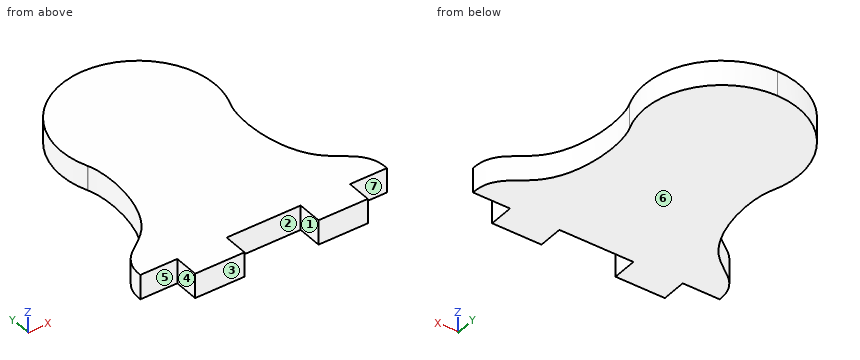
```python
from build123d import *

# Parameters (mm, degrees)
BOSS_EXTRUDE1_DEPTH = 4


with BuildPart() as part:
    # Sketch1 → Boss-Extrude1 (new body)
    with BuildSketch(Plane.XY):
        with BuildLine():
            Line((-6, 0), (0, 0))
            Line((0, 0), (0, 40.631746277))
            ThreePointArc((0, 40.631746277), (-10.364472675, 35.119428737), (-11.587783027, 23.444179263))
            ThreePointArc((-11.587783027, 23.444179263), (-11.580453389, 23.426100806), (-11.573095546, 23.40803381))
            add(Edge.make_bspline(
                [(-20, 0), (-20.119909127, 4.314498585), (-10.868715854, 6.603153145), (-10.177575907, 19.938030034), (-11.573095546, 23.40803381)],
                knots=[0, 0, 0, 0, 0.217805144, 0.603787586, 0.603787586, 0.603787586, 0.603787586], degree=3))
            Line((-20, 0), (-14, 0))
            Line((-14, 0), (-14, -4))
            Line((-14, -4), (-6, -4))
            Line((-6, -4), (-6, 0))
        make_face()
        with BuildLine():
            Line((0, 40.631746277), (0, 0))
            Line((0, 0), (6, 0))
            Line((6, 0), (6, -4))
            Line((6, -4), (14, -4))
            Line((14, -4), (14, 0))
            Line((14, 0), (20, 0))
            add(Edge.make_bspline(
                [(20, 0), (20.119909127, 4.314498585), (10.868715854, 6.603153145), (10.177575907, 19.938030034), (11.573095546, 23.40803381)],
                knots=[0, 0, 0, 0, 0.217805144, 0.603787586, 0.603787586, 0.603787586, 0.603787586], degree=3))
            ThreePointArc((11.573095546, 23.40803381), (11.580453389, 23.426100806), (11.587783027, 23.444179263))
            ThreePointArc((11.587783027, 23.444179263), (10.364472675, 35.119428737), (0, 40.631746277))
        make_face()
    extrude(amount=BOSS_EXTRUDE1_DEPTH)


solid = part.part
```
Input: part model. Units: mm. Frame: model coordinates. Face numbers are marked on the shaded views. A direction names the side the tool comes from. Coordinates: 2 decimals unless noted, no trailing zeros. Loops run counter-clockwise (first coordinate to the right, second up) from the corner with the lowest first, then second, coordinate; pieces in that order, holes last. Notation, with made-up numbers: M 67.25,62 L 114.25,62 A36 cw 114.25,97 Z; hole C 43,68 d3. An arc over 180 degrees is marked long. Use a Markdown table: item, result. Add a question column.
1) Section B-B, the plane x = -2. Return the cut outline in (y, z).
2) Set-up query: the marked faces 5, 6 and 7. Return all of +Z, -Z, +X, -X, +Y, -Y with unobstructed straight access to the full face (end or side cutting, diameter ignored); none if empty.
3) Line query: L1, parallel to X at y = 18.5, z = 3.8; L2, parallel to X at y = 28, z = 2.7; L3, parallel to Y at x = -1.5, z = 1.9. Output: solid intervals per line, ascending. Write a range as from..to.
4) Section A-A, the plane y = 37. Return the cut outline in (x, z).
5) Pin query (flat end, axial travel): P1, Ø2, axis at x = 2, z = 3.5, coming from the -Y side; P2, Ø1.2, axis at y = -2, z = 3, coming from the -X side; P3, Ø1.2, axis at y = -1.5, z = 3, coming from the +X side. Return the tip coordinate at first contact, or that it passes through.
6) Draft query along X for the marked faces 1, 2, 3 and 4. Return one class per face: +X half, -X half, draft (parallel to the pull), parting line (faces both ways), or undercut.
Answer below:
| question | item | result |
|---|---|---|
| 1 | outline | M 0,0 L 40.47,0 L 40.47,4 L 0,4 Z |
| 2 | face 5 | +Z, -Z, -X, -Y |
| 2 | face 6 | -Z, +X, -X, +Y, -Y |
| 2 | face 7 | +Z, -Z, +X, -Y |
| 3 | L1 | -10.85..10.85 |
| 3 | L2 | -12.5..12.5 |
| 3 | L3 | 0..40.54 |
| 4 | outline | M -8.81,0 L 8.81,0 L 8.81,4 L -8.81,4 Z |
| 5 | P1 | y = 0 |
| 5 | P2 | x = -14 |
| 5 | P3 | x = 14 |
| 6 | face 1 | undercut |
| 6 | face 2 | undercut |
| 6 | face 3 | draft |
| 6 | face 4 | -X half |
